Design review of the part shown in the three views and the two pictorial views. Dimensions are in mm from the part's minimum x, y and z. A direction names the side the tool comes from. Coordinates: 2 decimals unless noted, no trailing zeros. Loops run counter-clockwise (first coordinate to the right, second up) from the corner with the lowest first, then second, coordinate; pieces in that order, holes last. Notation, with made-up numbers: (68.5, -28.5) -> (124.5, -28.5) arc R28 cw to (124.5, -10.5) -> close; hole circle Ø4 at (-6, 7). An arc over 180 degrees is marked (long way). Answer in a Markdown table with one row per item.
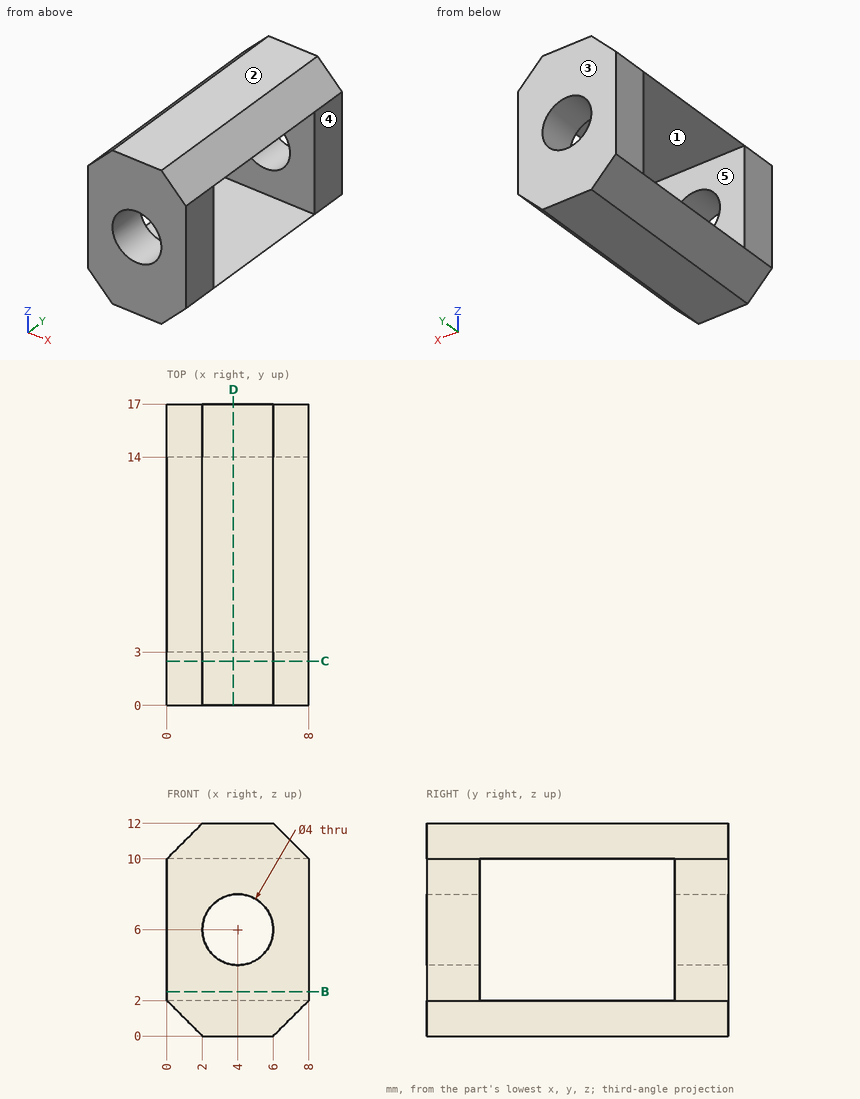
Item 1: Take a section at B-B, the plane z = 2.5. State the section outline as (x, y) points, and give its area (3 significant figures).
Worked answers:
| item | result |
|---|---|
| outline | (0, 0) -> (8, 0) -> (8, 3) -> (0, 3) -> close; (0, 14) -> (8, 14) -> (8, 17) -> (0, 17) -> close |
| area | 48.0 mm² |
Item 2: For the marked faces 4 and 5, list the 3-axis set-ups (+Z, -Z, +X, -X, +Y, -Y) from which the entire face can be reached by the end or side of a thin tool; tool diameter is ignored.
Worked answers:
| item | result |
|---|---|
| face 4 | +Z, -Z, +X, +Y, -Y |
| face 5 | +X, -X |
Item 3: Take a section at D-D, the plane x = 3.75. State the section outline as (y, z) points, and give its area (3 significant figures).
Worked answers:
| item | result |
|---|---|
| outline | (0, 0) -> (17, 0) -> (17, 4.02) -> (14, 4.02) -> (14, 2) -> (3, 2) -> (3, 4.02) -> (0, 4.02) -> close; (0, 7.98) -> (3, 7.98) -> (3, 10) -> (14, 10) -> (14, 7.98) -> (17, 7.98) -> (17, 12) -> (0, 12) -> close |
| area | 92.2 mm² |
Item 4: For L1, parallel to Y at x = 7, z = 2.5; L2, parallel to Z at x = 3.75, y = 6; L3, parallel to Z at x = 4, y = 1.3, list the stretches that pass through material, from the lowest coordinate up.
Worked answers:
| item | result |
|---|---|
| L1 | 0 to 3, 14 to 17 |
| L2 | 0 to 2, 10 to 12 |
| L3 | 0 to 4, 8 to 12 |
Item 5: The part is to be moulded in two halves that separate along Y. For the marked faces 1, 2 and 3, say which applies: +Y half, -Y half, draft (parallel to the pull), parting line (faces both ways), or undercut.
Worked answers:
| item | result |
|---|---|
| face 1 | undercut |
| face 2 | draft |
| face 3 | +Y half |
Item 6: Insertion check: pin 1 (3 mm diameter, centred on y = 11.5, z = 1.5, fed in from -X); pin 2 (1.5 mm diameter, centred on y = 5, z = 2.5, fed in from +X). Each pin has a flat end and moves straight along its axis. Give the tip position at first contact, or say it passes through.
Worked answers:
| item | result |
|---|---|
| pin 1 | x = 0 |
| pin 2 | x = 8 |
Item 7: Take a section at C-C, the plane y = 2.5. State the section outline as (x, z) points, and give its area (3 significant figures).
Worked answers:
| item | result |
|---|---|
| outline | (0, 2) -> (2, 0) -> (6, 0) -> (8, 2) -> (8, 10) -> (6, 12) -> (2, 12) -> (0, 10) -> close; hole circle Ø4 at (4, 6) |
| area | 75.4 mm² |
